Check sheet for the modelled part. Datum: model origin and axes. Units: mm. Face numbers are marked on the shaded views. Give positions to 0.01 mm unless a question says otherwise; leave off trailing zeros. Order: outer loops, then holes, each group sorted by start corner. A loop starts at its lowest first (then second) coordinate and runs counter-clockwise, first axis right, second up. Notation, with made-up numbers: (80, 51.25) - (127, 51.25) arc R18 ccw to (127, 65.25) - close; hole circle Ø1 at (82, -16). An arc over 180 degrees is marked (long way). Answer in a Markdown table with one row per item.
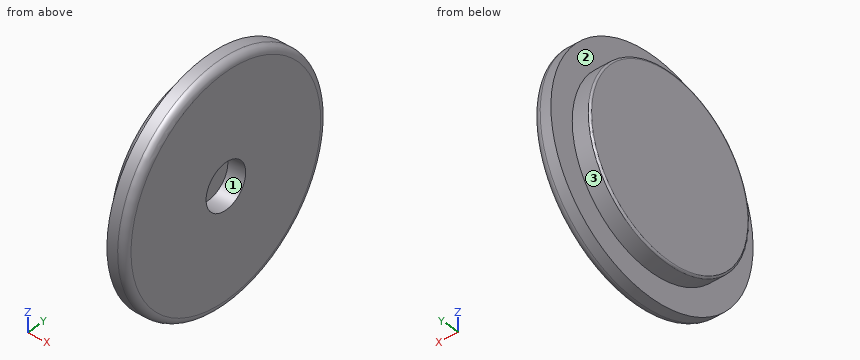
from build123d import *

# Parameters (mm, degrees)
SKETCH1_R           = 51.15
BOSS_EXTRUDE1_DEPTH = 10
SKETCH2_R           = 64.84855049
BOSS_EXTRUDE2_DEPTH = 10
SKETCH3_R           = 12.7
CUT_EXTRUDE1_DEPTH  = 10
FILLET1_R           = 1
FILLET2_R           = 4


with BuildPart() as part:
    # Sketch1 → Boss-Extrude1 (new body)
    with BuildSketch(Plane(origin=(0, 0, 0), x_dir=(0, 0, -1), z_dir=(1, 0, 0))):
        Circle(SKETCH1_R)
    extrude(amount=BOSS_EXTRUDE1_DEPTH)

    # Sketch2 → Boss-Extrude2 (add)
    with BuildSketch(Plane(origin=(10, 0, 0), x_dir=(0, 0, -1), z_dir=(1, 0, 0))):
        Circle(SKETCH2_R)
    extrude(amount=BOSS_EXTRUDE2_DEPTH)

    # Sketch3 → Cut-Extrude1 (cut)
    with BuildSketch(Plane(origin=(20, 0, 0), x_dir=(0, 0, -1), z_dir=(1, 0, 0))):
        Circle(SKETCH3_R)
    extrude(amount=-CUT_EXTRUDE1_DEPTH, mode=Mode.SUBTRACT)

    # Fillet1
    fillet1_edges = [part.edges().sort_by_distance(p)[0] for p in [
        (0, 0, 51.15),
    ]]
    fillet(fillet1_edges, radius=FILLET1_R)

    # Fillet2
    fillet2_edges = [part.edges().sort_by_distance(p)[0] for p in [
        (20, 0, 64.84855049),
    ]]
    fillet(fillet2_edges, radius=FILLET2_R)


solid = part.part
(1) Cross-section at A-A, the plane y = 0. Record the cut outline in (x, z).
Geometry says:
| item | result |
|---|---|
| outline | (0, -50.15) arc R1 ccw to (1, -51.15) - (10, -51.15) - (10, -64.85) - (16, -64.85) arc R4 ccw to (20, -60.85) - (20, -12.7) - (10, -12.7) - (10, 12.7) - (20, 12.7) - (20, 60.85) arc R4 ccw to (16, 64.85) - (10, 64.85) - (10, 51.15) - (1, 51.15) arc R1 ccw to (0, 50.15) - close |
(2) Mould release check, pull along Z, two halves, no side actions. Record for the marked faces 1, 2 and 3: pulls with the +Z half, pulls with the -Z half, needs draft (parallel to the pull), parting line crosses it, or undercut.
Geometry says:
| item | result |
|---|---|
| face 1 | undercut |
| face 2 | needs draft |
| face 3 | parting line crosses it |
(3) Cross-section at C-C, the plane x = 12. Record the cut outline in (y, z), then the cut area to 3 significant figures.
Geometry says:
| item | result |
|---|---|
| outline | circle Ø129.7 at (0, 0); hole circle Ø25.4 at (0, 0) |
| area | 12,700 mm² |
(4) Cross-section at D-D, the plane x = 2.75. Record the cut outline in (y, z), then the cut area to 3 significant figures.
Geometry says:
| item | result |
|---|---|
| outline | circle Ø102.3 at (0, 0) |
| area | 8,220 mm² |
(5) Thickness scan on L1, parallel to Y at x = 14.5, z = 0; L2, parallel to X at y = -40, z = 40; L3, parallel to Y at x = 17.5, z = 0. Record the ranges inside material, lowest first.
Geometry says:
| item | result |
|---|---|
| L1 | -64.85 to -12.7, 12.7 to 64.85 |
| L2 | 10 to 20 |
| L3 | -64.56 to -12.7, 12.7 to 64.56 |
(6) Gauge pin test, flat ends, axial feed: P1, Ø8, axis at x = 8, y = -10, coming from the -Z side; P2, Ø10, axis at x = 5.5, y = 28, coming from the -Z side; P3, Ø2, axis at x = 8.5, y = 37, coming from the -Z side. Record the tip position at first contact, or that the pin passes through.
Geometry says:
| item | result |
|---|---|
| P1 | z = -64.52 |
| P2 | z = -59.49 |
| P3 | z = -36.34 |
